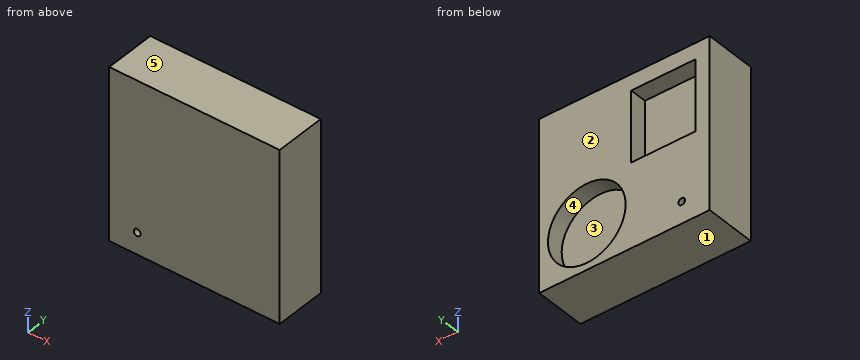
from build123d import *

# Parameters (mm, degrees)
SKETCH1_W           = 100
SKETCH1_H           = 100
BOSS_EXTRUDE1_DEPTH = 30
SKETCH5_R           = 2
CUT_EXTRUDE1_DEPTH  = 31
SKETCH7_R           = 22.78996388
SKETCH7_W           = 37.683489423
SKETCH7_H           = 41.413312703
CUT_EXTRUDE2_DEPTH  = 10


with BuildPart() as part:
    # Sketch1 → Boss-Extrude1 (new body)
    with BuildSketch(Plane(origin=(0, 0, 0), x_dir=(1, 0, 0), z_dir=(0, 1, 0))):
        with Locations((50, 50)):
            Rectangle(SKETCH1_W, SKETCH1_H)
    extrude(amount=BOSS_EXTRUDE1_DEPTH)

    # Sketch5 → Cut-Extrude1 (cut, through all)
    with BuildSketch(Plane(origin=(0, 30, 0), x_dir=(1, 0, 0), z_dir=(0, 1, 0))):
        with Locations((16.384313545, 87.323198024)):
            Circle(SKETCH5_R)
    extrude(amount=-CUT_EXTRUDE1_DEPTH, mode=Mode.SUBTRACT)

    # Sketch7 → Cut-Extrude2 (cut)
    with BuildSketch(Plane(origin=(0, 30, 0), x_dir=(1, 0, 0), z_dir=(0, 1, 0))):
        with Locations((72.084640228, 73.225170758)):
            Circle(SKETCH7_R)
        with Locations((27.16963915, 30.080771209)):
            Rectangle(SKETCH7_W, SKETCH7_H)
    extrude(amount=-CUT_EXTRUDE2_DEPTH, mode=Mode.SUBTRACT)


solid = part.part
The listing builds one solid part. Answer for the finished solid, in the listing's coordinates (mm). Face numbers are marked on the shaded views. A direction names the side the tool comes from. Give positions to 0.01 mm unless a question says otherwise; leave off trailing zeros. Write each loop counter-clockwise with the first axis right and the second up, starting at its lowest first coordinate (ties: lowest second). Pieces come first, ordered by that corner, then holes.
Item 1: Which of the six approach directions +Z, -Z, +X, -X, +Y, -Y give full straight-line access (tool end or side, diameter ignored) to the marked faces 4 and 5?
Item 2: Section C-C, the plane y = 27.5 is taken. Write down the section's boundary in (x, z), plus the area to 3 significant figures.
Item 3: Find the intervals of material crossed by line 1 along Z through (x, y) = (43, 21); line 2 along X through (y, z) = (22.5, -47); line 3 along X through (y, z) = (28, -73.5), in increasing order.
Item 4: Section B-B, the plane z = -11 is taken. Write down the section's boundary in (x, y), plus the area to 3 significant figures.
Item 5: Determine the mould class of the marked faces 1, 2 and 3 for opening direction Z: released by +Z, released by -Z, zero draft, split by the parting line, or undercut.
Item 6: Section A-A, the plane x = 20.5 is taken. Write down the section's boundary in (y, z).
Completed:
1. face 4: +Y
1. face 5: +Z, +X, -X, +Y, -Y
2. outline: (0, -100) - (100, -100) - (100, 0) - (0, 0) - close; hole (8.33, -50.79) - (46.01, -50.79) - (46.01, -9.37) - (8.33, -9.37) - close; hole circle Ø4 at (16.38, -87.32); hole circle Ø45.58 at (72.08, -73.23)
2. area: 6,800 mm2
3. line 1: z = -100 to -50.79, -9.37 to 0
3. line 2: x = 0 to 8.33, 46.01 to 100
3. line 3: x = 0 to 49.3, 94.87 to 100
4. outline: (0, 0) - (100, 0) - (100, 30) - (46.01, 30) - (46.01, 20) - (8.33, 20) - (8.33, 30) - (0, 30) - close
4. area: 2,620 mm2
5. face 1: released by -Z
5. face 2: zero draft
5. face 3: undercut
6. outline: (0, -100) - (30, -100) - (30, -50.79) - (20, -50.79) - (20, -9.37) - (30, -9.37) - (30, 0) - (0, 0) - close
